from build123d import *

# Parameters (mm, degrees)
SKETCH_1_R          = 10
SKETCH_1_R_2        = 9.128348481
EXTRUDE_2_DEPTH     = 1
SKETCH_1_4_R        = 9.128348481
EXTRUDE_4_DEPTH     = 10.5
SKETCH_1_5_R        = 1.1
CUT_EXTRUDE_1_DEPTH = 5


with BuildPart() as part:
    # 草图1 → 凸台-拉伸2 (new body)
    with BuildSketch(Plane(origin=(0, 0, 0), x_dir=(1, 0, 0), z_dir=(0, 1, 0))):
        Circle(SKETCH_1_R)
        Circle(SKETCH_1_R_2, mode=Mode.SUBTRACT)
    extrude(amount=EXTRUDE_2_DEPTH)

    # 草图1<4> → 凸台-拉伸4 (add)
    with BuildSketch(Plane(origin=(0, 0, 0), x_dir=(1, 0, 0), z_dir=(0, 1, 0))):
        Circle(SKETCH_1_4_R)
        with BuildLine():
            Line((0.473140602, 4.307795347), (0.473140602, 8.075783591))
            ThreePointArc((0.473140602, 8.075783591), (7.005826645, 4.044815899), (7.230404046, -3.628140015))
            Line((7.230404046, -3.628140015), (3.967230505, -1.744145892))
            ThreePointArc((3.967230505, -1.744145892), (3.753095001, 2.166850409), (0.473140602, 4.307795347))
        make_face(mode=Mode.SUBTRACT)
        with BuildLine():
            Line((-0.473140602, 8.075783591), (-0.473140602, 4.307795347))
            ThreePointArc((-0.473140602, 4.307795347), (-3.753095001, 2.166850409), (-3.967230505, -1.744145892))
            Line((-3.967230505, -1.744145892), (-7.230404046, -3.628140015))
            ThreePointArc((-7.230404046, -3.628140015), (-7.005826645, 4.044815899), (-0.473140602, 8.075783591))
        make_face(mode=Mode.SUBTRACT)
        with BuildLine():
            Line((-6.757263444, -4.447643576), (-3.494089903, -2.563649454))
            ThreePointArc((-3.494089903, -2.563649454), (0, -4.333700818), (3.494089903, -2.563649454))
            Line((3.494089903, -2.563649454), (6.757263444, -4.447643576))
            ThreePointArc((6.757263444, -4.447643576), (0, -8.089631799), (-6.757263444, -4.447643576))
        make_face(mode=Mode.SUBTRACT)
    extrude(amount=EXTRUDE_4_DEPTH)

    # 草图2 → 切除-旋转1 (revolve, cut)
    with BuildSketch(Plane(origin=(0, 0, 0), x_dir=(0, 0, -1), z_dir=(1, 0, 0))):
        with BuildLine():
            Line((8.099016848, 10.5), (8.099016848, 7.718955254))
            Line((8.099016848, 7.718955254), (4.307795347, 6.293437734))
            Line((4.307795347, 6.293437734), (3.916728598, 6.293437734))
            Line((3.916728598, 6.293437734), (3.916728598, 3.964130755))
            add(Edge.make_bspline(
                [(3.916728598, 3.964130755), (3.198487501, 5.366870317), (1.55626671, 6.233016223), (0, 6.17174819)],
                knots=[0, 0, 0, 0, 1, 1, 1, 1], degree=3))
            Line((0, 6.17174819), (0, 6.293437734))
            Line((0, 6.293437734), (0, 10.5))
            Line((0, 10.5), (8.099016848, 10.5))
        make_face()
    revolve(axis=Axis((0, 2.702728724, 0), (0, 1, 0)), mode=Mode.SUBTRACT)

    # 草图1<5> → 切除-拉伸1 (cut)
    with BuildSketch(Plane(origin=(0, 0, 0), x_dir=(1, 0, 0), z_dir=(0, 1, 0))):
        Circle(SKETCH_1_5_R)
    extrude(amount=CUT_EXTRUDE_1_DEPTH, mode=Mode.SUBTRACT)

    # 草图3 → 旋转1 (revolve)
    with BuildSketch(Plane(origin=(0, 0, 0), x_dir=(0, 0, -1), z_dir=(1, 0, 0))):
        with BuildLine():
            Line((1.1, 0), (1.1, -4))
            Line((1.1, -4), (1.858610419, -4))
            add(Edge.make_bspline(
                [(1.858610419, -4), (1.970625951, -1.457794417), (4.274857556, 0)],
                knots=[0, 0, 0, 1, 1, 1], degree=2))
            Line((4.274857556, 0), (1.1, 0))
        make_face()
    revolve(axis=Axis((0, -4.725, 0), (0, 1, 0)))


solid = part.part
The model under review builds one solid part; all positions refer to its coordinate system, in mm. A direction names the side the tool comes from. Round coordinates to 2 decimals unless told otherwise and drop trailing zeros. Write each loop counter-clockwise with the first axis right and the second up, starting at its lowest first coordinate (ties: lowest second). Pieces come first, ordered by that corner, then holes. Notation, with made-up numbers: (79, 89.5) - (133, 89.5) arc R28 cw to (133, 111.5) - close; hole circle Ø10 at (55.25, 81.25). An arc over 180 degrees is marked (long way). One line per item, written item: value. Start each with the question number.
1. Clearance check with flat-ended pins moving along their axes: P1, Ø8, axis at x = 8, y = 4.5, coming from the +Z side; P2, Ø2, axis at y = 5, z = 3, coming from the -X side; P3, Ø8, axis at x = 1, y = 6, coming from the +Z side. State where each tip first meets the part, or that it passes through.
2. Consider section A-A on y = 1.75. Write out the cut boundary in (x, z).
3. To check wall thickness, follow L1, parallel to Z at x = 0, y = 4.6; L2, parallel to Z at x = 0, y = 9.65. State the ranges of each line that lie inside material, in increasing order. Write a range as from..to.
4. Machinability: for faces 4 (the face through (1, -4, 1)), 5 (the face through (0, 5, 0)), 6 (the face through (0.473, 4, -6)), 7 (the face through (4, 6.293, -1)), which of the approach directions +Z, -Z, +X, -X, +Y, -Y give a long, thin tool a straight path to every point of the face, cutting with its end or side? Answer none if there is none.
5. The part is to be moulded in two halves that separate along Z. For faces 1 (the face through (6.95, 3.8, -4.14)), 2 (the face through (3, 1, 9)), 3 (the face through (-2.17, 0.49, 9.76)), say which applies: released by +Z, released by -Z, zero draft, split by the parting line, or undercut.
6. Consider section B-B on x = -5.5. State how many separate pieces and enclosed holes the cut face has, and give its area (3 significant figures).
Checks:
1. P1: stops at z = 8.21
1. P2: stops at x = -8.91
1. P3: stops at z = 9.13
2. outline: circle Ø18.26 at (0, 0); hole (-7.23, 3.63) arc R8.09 ccw to (-0.47, -8.08) - (-0.47, -4.31) arc R4.33 cw to (-3.97, 1.74) - close; hole (-6.76, 4.45) - (-3.49, 2.56) arc R4.33 cw to (3.49, 2.56) - (6.76, 4.45) arc R8.09 ccw to start; hole circle Ø2.2 at (0, 0); hole (0.47, -8.08) arc R8.09 ccw to (7.23, 3.63) - (3.97, 1.74) arc R4.33 cw to (0.47, -4.31) - close
3. L1: z = -9.13..-3.92, -3.5..-1.1, 1.1..3.5, 3.92..4.33, 8.09..9.13
3. L2: z = -9.13..-8.1, 8.1..9.13
4. face 4: +Z, -Z, +X, -X, -Y
4. face 5: -Y
4. face 6: +Y, -Y
4. face 7: +Y
5. face 1: undercut
5. face 2: zero draft
5. face 3: split by the parting line
6. separate pieces: 3
6. enclosed holes: 0
6. area: 38.2 mm^2
